```python
from build123d import *

# Parameters (mm, degrees)
ESBO_O1_W                   = 115
ESBO_O1_H                   = 200
RESSALTO_EXTRUS_O1_DEPTH    = 5
FURO_COM_FOLGA_DE_M41_D     = 4.5
ESBO_O5_W                   = 24
ESBO_O5_H                   = 5
CORTE_EXTRUS_O1_DEPTH       = 45
ESBO_O6_W                   = 24
ESBO_O6_H                   = 5
CORTE_EXTRUS_O2_DEPTH       = 45
ESBO_O7_W                   = 64.7
ESBO_O7_H                   = 51
CORTE_EXTRUS_O3_DEPTH       = 2.5
FURO_COM_FOLGA_DE_M31_D     = 3.4
ESBO_O10_W                  = 18
ESBO_O10_H                  = 19
CORTE_EXTRUS_O4_DEPTH       = 2.2
ESBO_O11_W                  = 10.5
ESBO_O11_H                  = 28
CORTE_EXTRUS_O5_DEPTH       = 231.759615184
FURO_COM_FOLGA_DE_M32_D     = 3.4
FURO_COM_FOLGA_DE_M33_D     = 3.4
FURO_COM_FOLGA_DE_M34_D     = 3.4
FURO_COM_FOLGA_DE_M35_D     = 3.4
FURO_COM_FOLGA_DE_M35_DEPTH = 11.25
FURO_COM_FOLGA_DE_M35_TIP   = 1.021463052
ESBO_O24_R                  = 2
CORTE_EXTRUS_O6_DEPTH       = 231.759615184
ESBO_O26_R                  = 2
CORTE_EXTRUS_O7_DEPTH       = 231.759615184
ESBO_O27_R                  = 2
CORTE_EXTRUS_O8_DEPTH       = 231.759615184


with BuildPart() as part:
    # Esboço1 → Ressalto-extrusão1 (new body)
    with BuildSketch(Plane(origin=(0, 0, 0), x_dir=(1, 0, 0), z_dir=(0, 1, 0))):
        with Locations((57.5, 100)):
            Rectangle(ESBO_O1_W, ESBO_O1_H)
    extrude(amount=RESSALTO_EXTRUS_O1_DEPTH)

    # Furo com folga de M41 (through all)
    with Locations(Plane(origin=(0, 5, 0), x_dir=(1, 0, 0), z_dir=(0, 1, 0))):
        with Locations((45.5, 5), (69.5, 5), (69.5, 35), (45.5, 35)):
            Hole(FURO_COM_FOLGA_DE_M41_D / 2)

    # Esboço5 → Corte-extrusão1 (cut)
    with BuildSketch(Plane.ZY):
        with Locations((-166.5, 2.5)):
            Rectangle(ESBO_O5_W, ESBO_O5_H)
    extrude(amount=-CORTE_EXTRUS_O1_DEPTH, mode=Mode.SUBTRACT)

    # Esboço6 → Corte-extrusão2 (cut)
    with BuildSketch(Plane(origin=(115, 0, 0), x_dir=(0, 0, -1), z_dir=(1, 0, 0))):
        with Locations((166.5, 2.5)):
            Rectangle(ESBO_O6_W, ESBO_O6_H)
    extrude(amount=-CORTE_EXTRUS_O2_DEPTH, mode=Mode.SUBTRACT)

    # Esboço7 → Corte-extrusão3 (cut)
    with BuildSketch(Plane(origin=(0, 5, 0), x_dir=(1, 0, 0), z_dir=(0, 1, 0))):
        with Locations((57.5, 80.5)):
            Rectangle(ESBO_O7_W, ESBO_O7_H)
    extrude(amount=-CORTE_EXTRUS_O3_DEPTH, mode=Mode.SUBTRACT)

    # Furo com folga de M31 (through all)
    with Locations(Plane(origin=(0, 5, 0), x_dir=(1, 0, 0), z_dir=(0, 1, 0))):
        with Locations((88.69, 61.62), (88.69, 89.56), (37.89, 104.8), (36.62, 56.54)):
            Hole(FURO_COM_FOLGA_DE_M31_D / 2)

    # Esboço10 → Corte-extrusão4 (cut)
    with BuildSketch(Plane(origin=(0, 5, 0), x_dir=(1, 0, 0), z_dir=(0, 1, 0))):
        with Locations((57.5, 135.5)):
            Rectangle(ESBO_O10_W, ESBO_O10_H)
    extrude(amount=-CORTE_EXTRUS_O4_DEPTH, mode=Mode.SUBTRACT)

    # Esboço11 → Corte-extrusão5 (cut, through all)
    with BuildSketch(Plane(origin=(0, 5, 0), x_dir=(1, 0, 0), z_dir=(0, 1, 0))):
        with Locations((13.25, 24)):
            Rectangle(ESBO_O11_W, ESBO_O11_H)
    extrude(amount=-CORTE_EXTRUS_O5_DEPTH, mode=Mode.SUBTRACT)

    # Furo com folga de M32 (through all)
    with Locations(Plane(origin=(0, 0, 0), x_dir=(-1, 0, 0), z_dir=(0, -1, 0))):
        with Locations((-15, 51.9), (-100, 51.9), (-100, 111.9), (-15, 111.9)):
            Hole(FURO_COM_FOLGA_DE_M32_D / 2)

    # Furo com folga de M33 (through all)
    with Locations(Plane(origin=(0, 5, 0), x_dir=(1, 0, 0), z_dir=(0, 1, 0))):
        with Locations((57.5, 153.7), (57.5, 117.3)):
            Hole(FURO_COM_FOLGA_DE_M33_D / 2)

    # Furo com folga de M34 (through all)
    with Locations(Plane(origin=(0, 5, 0), x_dir=(1, 0, 0), z_dir=(0, 1, 0))):
        with Locations((22.5, 186.95), (22.5, 146.05), (92.5, 186.95), (92.5, 146.05)):
            Hole(FURO_COM_FOLGA_DE_M34_D / 2)

    # Furo com folga de M35
    with Locations(Plane(origin=(0, 5, 0), x_dir=(1, 0, 0), z_dir=(0, 1, 0))):
        with Locations((76.2, 194), (38.8, 194)):
            Hole(FURO_COM_FOLGA_DE_M35_D / 2, depth=FURO_COM_FOLGA_DE_M35_DEPTH)
            with Locations((0, 0, -(FURO_COM_FOLGA_DE_M35_DEPTH + FURO_COM_FOLGA_DE_M35_TIP / 2))):  # 118° drill point
                Cone(0, FURO_COM_FOLGA_DE_M35_D / 2, FURO_COM_FOLGA_DE_M35_TIP, mode=Mode.SUBTRACT)

    # Esboço24 → Corte-extrusão6 (cut, through all)
    with BuildSketch(Plane(origin=(0, 5, 0), x_dir=(1, 0, 0), z_dir=(0, 1, 0))):
        with Locations(Location((45, 148, 0), (0, 0, 270))):
            Circle(ESBO_O24_R)
        with Locations(Location((50, 148, 0), (0, 0, 270))):
            Circle(ESBO_O24_R)
        with Locations(Location((65, 148, 0), (0, 0, 270))):
            Circle(ESBO_O24_R)
        with Locations(Location((70, 148, 0), (0, 0, 270))):
            Circle(ESBO_O24_R)
        with Locations(Location((70, 143, 0), (0, 0, 270))):
            Circle(ESBO_O24_R)
        with Locations(Location((70, 138, 0), (0, 0, 270))):
            Circle(ESBO_O24_R)
        with Locations(Location((70, 133, 0), (0, 0, 270))):
            Circle(ESBO_O24_R)
        with Locations(Location((70, 128, 0), (0, 0, 270))):
            Circle(ESBO_O24_R)
        with Locations(Location((70, 123, 0), (0, 0, 270))):
            Circle(ESBO_O24_R)
        with Locations(Location((65, 123, 0), (0, 0, 270))):
            Circle(ESBO_O24_R)
        with Locations(Location((50, 123, 0), (0, 0, 270))):
            Circle(ESBO_O24_R)
        with Locations(Location((45, 123, 0), (0, 0, 270))):
            Circle(ESBO_O24_R)
        with Locations(Location((45, 128, 0), (0, 0, 270))):
            Circle(ESBO_O24_R)
        with Locations(Location((45, 133, 0), (0, 0, 270))):
            Circle(ESBO_O24_R)
        with Locations(Location((45, 138, 0), (0, 0, 270))):
            Circle(ESBO_O24_R)
        with Locations(Location((45, 143, 0), (0, 0, 270))):
            Circle(ESBO_O24_R)
    extrude(amount=-CORTE_EXTRUS_O6_DEPTH, mode=Mode.SUBTRACT)

    # Esboço26 → Corte-extrusão7 (cut, through all)
    with BuildSketch(Plane(origin=(0, 5, 0), x_dir=(1, 0, 0), z_dir=(0, 1, 0))):
        with Locations(Location((46.35, 111, 0), (0, 0, 270))):
            Circle(ESBO_O26_R)
        with Locations(Location((51.35, 111, 0), (0, 0, 270))):
            Circle(ESBO_O26_R)
        with Locations(Location((61.35, 111, 0), (0, 0, 270))):
            Circle(ESBO_O26_R)
        with Locations(Location((66.35, 111, 0), (0, 0, 270))):
            Circle(ESBO_O26_R)
        with Locations(Location((71.35, 111, 0), (0, 0, 270))):
            Circle(ESBO_O26_R)
        with Locations(Location((81.35, 111, 0), (0, 0, 270))):
            Circle(ESBO_O26_R)
        with Locations(Location((86.35, 111, 0), (0, 0, 270))):
            Circle(ESBO_O26_R)
        with Locations(Location((56.35, 111, 0), (0, 0, 270))):
            Circle(ESBO_O26_R)
        with Locations(Location((76.35, 111, 0), (0, 0, 270))):
            Circle(ESBO_O26_R)
    extrude(amount=-CORTE_EXTRUS_O7_DEPTH, mode=Mode.SUBTRACT)

    # Esboço27 → Corte-extrusão8 (cut, through all)
    with BuildSketch(Plane(origin=(0, 5, 0), x_dir=(1, 0, 0), z_dir=(0, 1, 0))):
        with Locations(Location((92, 50, 0), (0, 0, 270))):
            Circle(ESBO_O27_R)
        with Locations(Location((82, 50, 0), (0, 0, 270))):
            Circle(ESBO_O27_R)
        with Locations(Location((67, 50, 0), (0, 0, 270))):
            Circle(ESBO_O27_R)
        with Locations(Location((77, 50, 0), (0, 0, 270))):
            Circle(ESBO_O27_R)
        with Locations(Location((72, 50, 0), (0, 0, 270))):
            Circle(ESBO_O27_R)
        with Locations(Location((87, 50, 0), (0, 0, 270))):
            Circle(ESBO_O27_R)
    extrude(amount=-CORTE_EXTRUS_O8_DEPTH, mode=Mode.SUBTRACT)


solid = part.part
```
CAD build for the part. Positions are in the model's coordinates, mm. A direction names the side the tool comes from. Round coordinates to 2 decimals unless told otherwise and drop trailing zeros. Order: outer loops, then holes, each group sorted by start corner. A loop starts at its lowest first (then second) coordinate and runs counter-clockwise, first axis right, second up. Notation, with made-up numbers: (-32.5, 70.25) - (20.5, 70.25) arc R14 ccw to (20.5, 85.25) - close; hole circle Ø1 at (18.25, 53.25). An arc over 180 degrees is marked (long way). Answer in a Markdown table with one row per item. Add a question column.
(1) Drop a flat-ended pin along its axis: pin 1 Ø2.5 at (x, z) = (50, -148) entering from -Y. Give the stop position or say it passes through.
(2) Band-saw the part on B-B on z = -164. List the corners of the cut face in (x, y).
(3) Band-saw the part on A-A on z = -24. List the corners of the cut face in (x, y).
(4) Probe L1, parallel to Z at x = 8.5, y = 0.85; L2, parallel to X at y = 3.8, z = -128; L3, parallel to Z at x = 63.5, y = 2.3. List the from-to ranges inside material, lowest first. Write a range as [from, to].
(5) Mould opens along Z. For faces 1 (the face through (55.133, 2.535, -112.587)), 2 (the face through (57, 2, -200)), 3 (the face through (45, 3, -167)), 4 (the face through (57, 0, -101)) say: +Z half, -Z half, draft (parallel to the pull), parting line (faces both ways), or undercut.
(6) 3-axis set-ups, long thin cutter, end or side, ignore diameter. For faces 5 (the face through (115, 2, -76)), 6 (the face through (0, 2, -189)), 7 (the face through (13, 3, -10)), 8 (the face through (22, 2, -154.5)), 9 (the face through (93, 2, -154.5)): which of +Z, -Z, +X, -X, +Y, -Y reach the whole face in a straight line?
Data:
| question | item | result |
|---|---|---|
| 1 | pin 1 | passes through |
| 2 | outline | (45, 0) - (70, 0) - (70, 5) - (45, 5) - close |
| 3 | outline | (0, 0) - (8, 0) - (8, 5) - (0, 5) - close; (18.5, 0) - (115, 0) - (115, 5) - (18.5, 5) - close |
| 4 | L1 | z = [-200, -178.5], [-154.5, -38], [-10, 0] |
| 4 | L2 | x = [0, 43], [47, 48.5], [66.5, 68], [72, 115] |
| 4 | L3 | z = [-200, -149.32], [-146.68, -124.32], [-121.68, 0] |
| 5 | face 1 | undercut |
| 5 | face 2 | -Z half |
| 5 | face 3 | undercut |
| 5 | face 4 | draft |
| 6 | face 5 | +Z, -Z, +X, +Y, -Y |
| 6 | face 6 | +Z, -Z, -X, +Y, -Y |
| 6 | face 7 | +Y, -Y |
| 6 | face 8 | -X, +Y, -Y |
| 6 | face 9 | +X, +Y, -Y |
